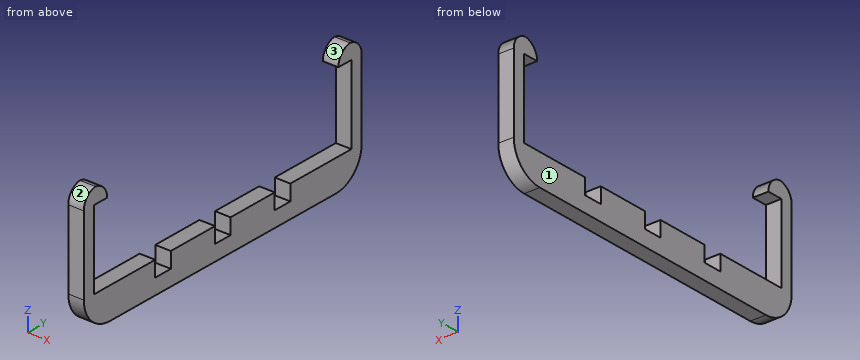
from build123d import *

# Parameters (mm, degrees)
F0_W         = 5
F0_H         = 107
F1_DEPTH     = 10
F3_W         = 5
F3_H         = 6
F4_DEPTH     = 5
F5_DEPTH     = 5
F6_R         = 9.99999
F2_W         = 5
F2_H         = 4
F7_DEPTH     = 30
F8_DEPTH     = 30
F9_W         = 5
F9_H         = 5
F10_DEPTH    = 5
F11_W        = 5
F11_H        = 5
F12_DEPTH    = 5
F13_T1_DEPTH = 30
F14_W        = 5
F14_H        = 6
F15_DEPTH    = 5


# Not quite as in the source:
# - a fillet or chamfer that OpenCascade refuses, or shapes differently, is made with other operations: its cross-section is extruded or revolved along the edge and cut away or added
# - a fillet or chamfer is up to 0.001 mm smaller than in the source, because OpenCascade refuses the exact size
# - a feature names something its author has since deleted; it is built from what else it names


with BuildPart() as f1:
    # F0 (on Top) → F1 (new body)
    with BuildSketch(Plane.XY):
        Rectangle(F0_W, F0_H)
    extrude(amount=F1_DEPTH)

    # F3 (on face) → F4 (cut)
    with BuildSketch(Plane.XY.offset(10)):
        with Locations((0, 23)):
            Rectangle(F3_W, F3_H)
    extrude(amount=-F4_DEPTH, mode=Mode.SUBTRACT)

    # F3 (on face) → F5 (cut)
    with BuildSketch(Plane.XY.offset(10)):
        with Locations((0, 23)):
            Rectangle(F3_W, F3_H)
        with Locations((0, -23)):
            Rectangle(F3_W, F3_H)
    extrude(amount=-F5_DEPTH, mode=Mode.SUBTRACT)

    # F6 (radius 10 in the source; OpenCascade refuses exactly that, so slightly less here)
    f6_edges = [f1.edges().sort_by_distance(p)[0] for p in [
        (0, -53.5, 0),
        (0, 53.5, 0),
    ]]
    fillet(f6_edges, radius=F6_R)

    # F2 (on face) → F7 (join)
    with BuildSketch(Plane.XY.offset(10)):
        with Locations((0, 51.5)):
            Rectangle(F2_W, F2_H)
    extrude(amount=F7_DEPTH)

    # F2 (on face) → F8 (join)
    with BuildSketch(Plane.XY.offset(10)):
        with Locations((0, 51.5)):
            Rectangle(F2_W, F2_H)
        with Locations((0, -51.5)):
            Rectangle(F2_W, F2_H)
    extrude(amount=F8_DEPTH)

    # F9 (on face) → F10 (join)
    with BuildSketch(Plane(origin=(0, -49.5, 0), x_dir=(-1, 0, 0), z_dir=(0, 1, 0))):
        with Locations((0, 37.5)):
            Rectangle(F9_W, F9_H)
    extrude(amount=F10_DEPTH)

    # F11 (on face) → F12 (join)
    with BuildSketch(Plane.XZ.offset(-49.5)):
        with Locations((0, 37.5)):
            Rectangle(F11_W, F11_H)
    extrude(amount=F12_DEPTH)

    # F13: fillet of radius 5 on 4 edges, made by hand

    # F13_s2 → F13_t1 (cut)
    with BuildSketch(Plane.YZ.offset(-15)):
        with BuildLine():
            ThreePointArc((-48.5, 40), (-52.0355339059, 38.5355339059), (-53.5, 35))
            Line((-53.5, 35), (-53.5, 40))
            Line((-53.5, 40), (-48.5, 40))
        make_face()
        with BuildLine():
            ThreePointArc((53.5, 35), (52.0355339059, 38.5355339059), (48.5, 40))
            Line((48.5, 40), (53.5, 40))
            Line((53.5, 40), (53.5, 35))
        make_face()
        with BuildLine():
            ThreePointArc((49.5, 40), (45.9644660941, 38.5355339059), (44.5, 35))
            Line((44.5, 35), (44.5, 40))
            Line((44.5, 40), (49.5, 40))
        make_face()
        with BuildLine():
            ThreePointArc((-44.5, 35), (-45.9644660941, 38.5355339059), (-49.5, 40))
            Line((-49.5, 40), (-44.5, 40))
            Line((-44.5, 40), (-44.5, 35))
        make_face()
    extrude(amount=F13_T1_DEPTH, mode=Mode.SUBTRACT)

    # F14 (on face) → F15 (cut)
    with BuildSketch(Plane.XY.offset(10)):
        Rectangle(F14_W, F14_H)
    extrude(amount=-F15_DEPTH, mode=Mode.SUBTRACT)


solid = f1.part
Geometry check sheet. Reference: the model listing, model coordinates, mm. Face numbers are marked on the shaded views. Coordinates: 2 decimals unless noted, no trailing zeros. Loops run counter-clockwise (first coordinate to the right, second up) from the corner with the lowest first, then second, coordinate; pieces in that order, holes last. Notation, with made-up numbers: (-2, 54.25) - (4, 54.25) arc R6 cw to (4, 63.25) - close; hole circle Ø10 at (79, -32). An arc over 180 degrees is marked (long way). Use one line per item in the form item = value. Start each with the question number.
Item 1: Section check B-B, the plane x = 0.25. Enter the section's corners in (y, z).
Item 2: Section check A-A, the plane z = 15. Enter the section's corners in (x, y).
Item 3: Section check D-D, the plane y = 11.5. Enter the section's corners in (x, z), and give its area (3 significant figures).
Item 4: Mould release check, pull along Y, two halves, no side actions. Record for the marked faces 1, 2 and 3: +Y half, -Y half, draft (parallel to the pull), parting line (faces both ways), or undercut.
Item 5: Section check C-C, the plane z = 9. Enter the section's corners in (x, y).
Item 6: Gauge pin test, flat ends, axial feed: pin 1 (2.5 mm diameter, centred on x = -0.5, y = 35, fed in from +Z); pin 2 (1.5 mm diameter, centred on x = 0.5, y = -46, fed in from -Z); pin 3 (1.5 mm diameter, centred on x = -1, z = 7, fed in from -Y); pin 4 (10 mm diameter, centred on y = -14, z = 11.5, fed in from -X). Record the tip position at first contact, or that the pin passes through.
Item 7: Thickness scan on probe 1 along Y at (x, z) = (0, 9.5); probe 2 along Y at (x, z) = (-1.25, 22); probe 3 along Z at (x, y) = (-2.2, -0.5). Record the ranges inside material, lowest first.
Computed:
q1.outline = (-53.5, 10) arc R10 ccw to (-43.5, 0) - (43.5, 0) arc R10 ccw to (53.5, 10) - (53.5, 35) arc R5 ccw to (49, 39.97) arc R5 ccw to (44.5, 35) - (49.5, 35) - (49.5, 10) - (26, 10) - (26, 5) - (20, 5) - (20, 10) - (3, 10) - (3, 5) - (-3, 5) - (-3, 10) - (-20, 10) - (-20, 5) - (-26, 5) - (-26, 10) - (-49.5, 10) - (-49.5, 35) - (-44.5, 35) arc R5 ccw to (-49, 39.97) arc R5 ccw to (-53.5, 35) - close
q2.outline = (-2.5, -53.5) - (2.5, -53.5) - (2.5, -49.5) - (-2.5, -49.5) - close; (-2.5, 49.5) - (2.5, 49.5) - (2.5, 53.5) - (-2.5, 53.5) - close
q3.outline = (-2.5, 0) - (2.5, 0) - (2.5, 10) - (-2.5, 10) - close
q3.area = 50.0 mm2
q4.face_1 = draft
q4.face_2 = -Y half
q4.face_3 = undercut
q5.outline = (-2.5, -53.45) - (2.5, -53.45) - (2.5, -26) - (-2.5, -26) - close; (-2.5, -20) - (2.5, -20) - (2.5, -3) - (-2.5, -3) - close; (-2.5, 3) - (2.5, 3) - (2.5, 20) - (-2.5, 20) - close; (-2.5, 26) - (2.5, 26) - (2.5, 53.45) - (-2.5, 53.45) - close
q6.pin_1 = 10
q6.pin_2 = 0.15
q6.pin_3 = -53.24
q6.pin_4 = -2.5
q7.probe_1 = -53.49 to -26, -20 to -3, 3 to 20, 26 to 53.49
q7.probe_2 = -53.5 to -49.5, 49.5 to 53.5
q7.probe_3 = 0 to 5
